```python
from build123d import *

# Parameters (mm, degrees)
F1_DEPTH = 11.43
F2_R     = 5.08


with BuildPart() as f1:
    # F0 (on Right) → F1 (new body)
    with BuildSketch(Plane.YZ):
        Polygon((0, 14.58829), (-62.113028, 14.58829), (-62.113028, 4.662237), (12.783553, 4.662237), (12.783553, 45.268815), (0, 45.268815), align=None)
    extrude(amount=F1_DEPTH)

    # F2
    f2_edges = [f1.edges().sort_by_distance(p)[0] for p in [
        (11.43, 0, 29.928552),
        (0, 0, 29.928552),
        (11.43, 12.783553, 24.965526),
        (11.43, -24.664737, 4.662237),
        (0, -24.664737, 4.662237),
        (0, 12.783553, 24.965526),
        (0, -62.113028, 9.625264),
        (11.43, -62.113028, 9.625264),
        (5.715, -62.113028, 4.662237),
        (5.715, 12.783553, 4.662237),
    ]]
    fillet(f2_edges, radius=F2_R)


solid = f1.part
```
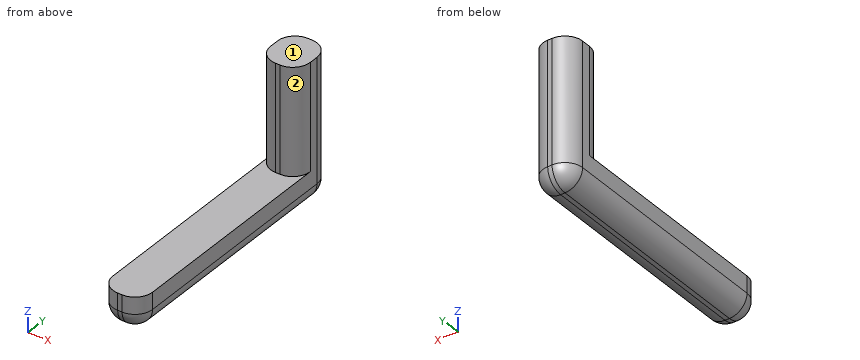
Geometry: final body of the model. Coordinates: model frame, mm. Face numbers are marked on the shaded views. A direction names the side the tool comes from. Round coordinates to 2 decimals unless told otherwise and drop trailing zeros. Order: outer loops, then holes, each group sorted by start corner. A loop starts at its lowest first (then second) coordinate and runs counter-clockwise, first axis right, second up. Notation, with made-up numbers: (52.25, 88.25) -> (103.25, 88.25) arc R21 cw to (103.25, 115.25) -> close; hole circle Ø1 at (10.25, -21.5). An arc over 180 degrees is marked (long way). Use one line per item in the form item = value. Start each with the question number.
1. Reachability of the marked faces 1 and 2 from +Z, -Z, +X, -X, +Y, -Y: full face, straight path, thin tool, end or side. Return the list, or none.
2. Line query: probe 1 along X at (y, z) = (5, 16.5); probe 2 along Y at (x, z) = (6.5, 10); probe 3 along Z at (x, y) = (5, -30.5). Output: solid intervals per line, ascending.
3. Cut plane C-C (y = -54). Return the cut outline in (x, z), then the cut area to 3 significant figures.
4. Cut plane A-A (z = 35). Return the cut outline in (x, y), then the cut area to 3 significant figures.
5. Cut plane B-B (x = 4). Return the cut outline in (y, z).
6. Pin query (flat end, axial travel): pin 1 Ø1.5 at (x, z) = (4, 19.5) entering from +Y; pin 2 Ø5.5 at (x, y) = (5, -34) entering from +Z; pin 3 Ø1.4 at (x, z) = (5.5, 28.5) entering from -Y. Return the tip coordinate at first contact, or that it passes through.
Solution:
q1.face_1 = +Z, +X, -X, +Y, -Y
q1.face_2 = +Z, +X, -Y
q2.probe_1 = 0 to 11.43
q2.probe_2 = -62.11 to 12.78
q2.probe_3 = 4.66 to 14.59
q3.outline = (0, 9.74) arc R5.08 ccw to (5.08, 4.66) -> (6.35, 4.66) arc R5.08 ccw to (11.43, 9.74) -> (11.43, 14.59) -> (0, 14.59) -> close
q3.area = 102 mm^2
q4.outline = (0, 5.08) arc R5.08 ccw to (5.08, 0) -> (6.35, 0) arc R5.08 ccw to (11.43, 5.08) -> (11.43, 7.7) arc R5.08 ccw to (6.35, 12.78) -> (5.08, 12.78) arc R5.08 ccw to (0, 7.7) -> close
q4.area = 124 mm^2
q5.outline = (-62, 9.74) arc R4.96 ccw to (-57.03, 4.78) -> (7.7, 4.78) arc R4.96 ccw to (12.67, 9.74) -> (12.67, 45.27) -> (0.12, 45.27) -> (0.12, 14.59) -> (-62, 14.59) -> close
q6.pin_1 = 12.77
q6.pin_2 = 14.59
q6.pin_3 = 0
